Drawing for the job (mm, zero at the part's lowest x, y, z). A direction names the side the tool comes from. Give positions to 0.01 mm unless a question says otherwise; leave off trailing zeros. Order: outer loops, then holes, each group sorted by start corner. A loop starts at its lowest first (then second) coordinate and runs counter-clockwise, first axis right, second up. Notation, with made-up numbers: (-34.75, 49.25) - (-8.75, 49.25) arc R20 ccw to (-8.75, 85.25) - close; hole circle Ø5 at (-33, -27.5). An arc over 180 degrees is marked (long way). One line per item, written item: value.
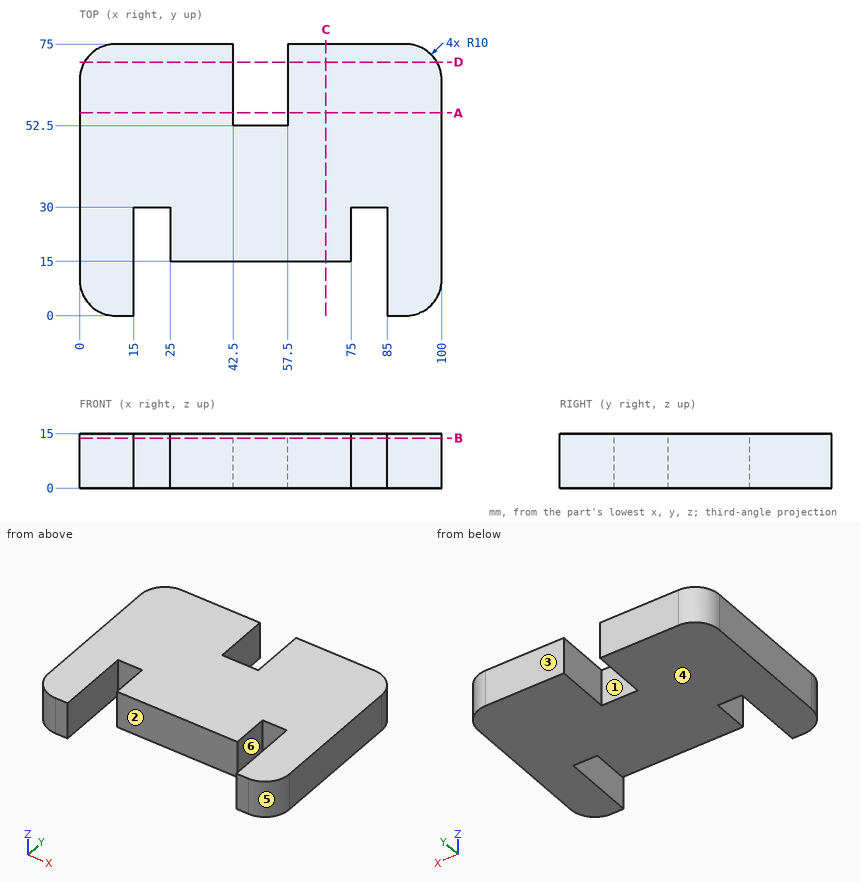
(1) Slice it at B-B, the plane z = 13.75. Give the cut face in (x, y), and give its area (3 significant figures).
Completed:
outline: (0, 10) arc R10 ccw to (10, 0) - (15, 0) - (15, 30) - (25, 30) - (25, 15) - (75, 15) - (75, 30) - (85, 30) - (85, 0) - (90, 0) arc R10 ccw to (100, 10) - (100, 65) arc R10 ccw to (90, 75) - (57.5, 75) - (57.5, 52.5) - (42.5, 52.5) - (42.5, 75) - (10, 75) arc R10 ccw to (0, 65) - close
area: 5,730 mm²
(2) Slice it at D-D, the plane y = 70. Give the cut face in (x, z), and give its area (3 significant figures).
Completed:
outline: (1.34, 0) - (42.5, 0) - (42.5, 15) - (1.34, 15) - close; (57.5, 0) - (98.66, 0) - (98.66, 15) - (57.5, 15) - close
area: 1,230 mm²
(3) 3-axis set-ups, long thin cutter, end or side, ignore diameter. For the marked faces 1, 2 and 3: which of +Z, -Z, +X, -X, +Y, -Y reach the whole face in a straight line?
Completed:
face 1: +Z, -Z, +Y
face 2: +Z, -Z, -Y
face 3: +Z, -Z, +X, -X, +Y
(4) Pin check, flat tip, straight feed: P1, Ø5, axis at x = 78.5, z = 8, coming from the -Y side. Stop position of the tip, or through.
Completed:
P1: y = 30
(5) Drill centre lines: line 1 (X direction, y = 28.5, z = 4); line 2 (X direction, y = 54, z = 14.25); line 3 (Y direction, x = 62, z = 2.5). Where is each one in solid material? Low to high.
Completed:
line 1: 0 to 15, 25 to 75, 85 to 100
line 2: 0 to 42.5, 57.5 to 100
line 3: 15 to 75
(6) Slice it at C-C, the plane x = 68. Give the cut face in (y, z), and give its area (3 significant figures).
Completed:
outline: (15, 0) - (75, 0) - (75, 15) - (15, 15) - close
area: 900 mm²
(7) Slice it at A-A, the plane y = 56. Give the cut face in (x, z), and give its area (4 significant figures).
Completed:
outline: (0, 0) - (42.5, 0) - (42.5, 15) - (0, 15) - close; (57.5, 0) - (100, 0) - (100, 15) - (57.5, 15) - close
area: 1,275 mm²
(8) Pull direction X, two halves, no side cores. Call the marked faces 4, 5 and 6: +X half, -X half, draft (parallel to the pull), parting line (faces both ways), or undercut.
Completed:
face 4: draft
face 5: +X half
face 6: undercut
